```python
from build123d import *

# Parameters (mm, degrees)
BOSS_EXTRUDE1_DEPTH     = 3
CUT_EXTRUDE1_DEPTH      = 14.421065531
CUT_EXTRUDE1_DEPTH_BACK = 14.421065531
SKETCH2_R               = 1.75
SKETCH3_R               = 4
CUT_EXTRUDE2_DEPTH      = 6
FILLET1_R               = 0.4
FILLET2_R               = 1
CUT_EXTRUDE3_DEPTH      = 15.391838135
CUT_EXTRUDE3_DEPTH_BACK = 15.391838135
SKETCH4_W               = 19
SKETCH4_H               = 0.4


with BuildPart() as part:
    # Sketch1 → Boss-Extrude1 (new, symmetric)
    with BuildSketch(Plane(origin=(0, 0, 0), x_dir=(1, 0, 0), z_dir=(0, 1, 0))):
        with BuildLine():
            Line((-4.05, 0), (-9.25, 0))
            ThreePointArc((-9.25, 0), (0, 9.25), (9.25, 0))
            Line((9.25, 0), (4.05, 0))
            ThreePointArc((4.05, 0), (0, 4.05), (-4.05, 0))
        make_face()
    extrude(amount=BOSS_EXTRUDE1_DEPTH, both=True)

    # Sketch2 → Cut-Extrude1 (cut, two sides: drawn at the far end of the back side and taken through both)
    with BuildSketch(Plane.XY.offset(-CUT_EXTRUDE1_DEPTH_BACK)):
        with Locations((6.65, 0)):
            Circle(SKETCH2_R)
        with Locations((-6.65, 0)):
            Circle(SKETCH2_R)
    extrude(amount=CUT_EXTRUDE1_DEPTH + CUT_EXTRUDE1_DEPTH_BACK, mode=Mode.SUBTRACT)

    # Sketch3 → Cut-Extrude2 (cut)
    with BuildSketch(Plane.XY.offset(-10)):
        with Locations((6.65, 0)):
            Circle(SKETCH3_R)
        with Locations((-6.65, 0)):
            Circle(SKETCH3_R)
    extrude(amount=CUT_EXTRUDE2_DEPTH, mode=Mode.SUBTRACT)

    # Fillet1
    # the kernel refuses this fillet: 0.4 mm, written as the material it takes off along each edge
    with BuildSketch(Plane(origin=(-4.004248689, 3, -4), x_dir=(0.6743792283231849, -0.7383851680567708, 0), z_dir=(0, 0, -1)), Plane(origin=(4.004248689, -3, -4), x_dir=(-0.6743792283231826, 0.7383851680567729, 0), z_dir=(0, 0, -1))) as fillet1_piece_1:
        with BuildLine():
            CenterArc((0.904923131, -0.397672121), FILLET1_R, 96.184415635, 126.22154662)
            Line((0.609569064, -0.667423812), (0, 0))
            ThreePointArc((0, 0), (0.430915777, -0.023278789), (0.861831553, 0))
        make_face()
    extrude(amount=6.598116085, mode=Mode.SUBTRACT)
    with BuildSketch(Plane(origin=(-4.004248689, -3, -4), x_dir=(0.6743792283231809, 0.7383851680567743, 0), z_dir=(0, 0, -1)), Plane(origin=(4.004248689, 3, -4), x_dir=(-0.6743792283231826, -0.7383851680567729, 0), z_dir=(0, 0, -1))) as fillet1_piece_2:
        with BuildLine():
            CenterArc((0.904923131, 0.397672121), FILLET1_R, 137.594037745, 126.22154662)
            Line((0.609569064, 0.667423812), (0, 0))
            ThreePointArc((0, 0), (0.430915777, 0.023278789), (0.861831553, 0))
        make_face()
    extrude(amount=6.598116085, mode=Mode.SUBTRACT)

    # Fillet2
    # the kernel refuses this fillet: 1 mm, written as the material it adds along each edge
    with BuildSketch(Plane(origin=(-6.65, 0, -4), x_dir=(0.8067381522408935, -0.5909090909090408, 0), z_dir=(-0.5909090909090408, -0.8067381522408935, 0))) as fillet2_piece_1:
        with BuildLine():
            CenterArc((4 - FILLET2_R, -FILLET2_R), FILLET2_R, 0, 90)
            Line((4, -FILLET2_R), (4, 0))
            Line((4, 0), (4 - FILLET2_R, 0))
        make_face()
    revolve(axis=Axis((-6.65, 0, -4), (0, 0, 1)), revolution_arc=72.44309324)
    with BuildSketch(Plane(origin=(6.65, 0, -4), x_dir=(-0.8067381522408924, 0.5909090909090423, 0), z_dir=(0.5909090909090423, 0.8067381522408924, 0))) as fillet2_piece_2:
        with BuildLine():
            CenterArc((4 - FILLET2_R, -FILLET2_R), FILLET2_R, 0, 90)
            Line((4, -FILLET2_R), (4, 0))
            Line((4, 0), (4 - FILLET2_R, 0))
        make_face()
    revolve(axis=Axis((6.65, 0, -4), (0, 0, 1)), revolution_arc=72.44309324)
    with BuildSketch(Plane(origin=(-3.10035213, 2.6, -4), x_dir=(-0.8067381522410291, -0.5909090909088556, 0), z_dir=(0.5909090909088556, -0.8067381522410291, 0))) as fillet2_piece_3_section:
        with BuildLine():
            CenterArc((0.4 + FILLET2_R, FILLET2_R), FILLET2_R, 180, 90)
            Line((0.4, FILLET2_R), (0.4, 0))
            Line((0.4, 0), (0.4 + FILLET2_R, 0))
        make_face()
    fillet2_piece_3 = revolve(axis=Axis((-3.10035213, 2.6, -4), (0, 0, -1)), revolution_arc=359.64, mode=Mode.PRIVATE)
    fillet2_piece_3 = split(fillet2_piece_3, bisect_by=Plane(origin=(-3.794786047, 3, -4.154806291), z_dir=(0, -1, 0)), keep=Keep.TOP, mode=Mode.PRIVATE)
    add(fillet2_piece_3)
    with BuildSketch(Plane(origin=(-3.10035213, -2.6, -4), x_dir=(-0.8030094610318433, 0.5959662788223411, 0), z_dir=(-0.5959662788223411, -0.8030094610318433, 0))) as fillet2_piece_4_section:
        with BuildLine():
            CenterArc((-0.4 - FILLET2_R, FILLET2_R), FILLET2_R, 270, 90)
            Line((-0.4 - FILLET2_R, 0), (-0.4, 0))
            Line((-0.4, 0), (-0.4, FILLET2_R))
        make_face()
    fillet2_piece_4 = revolve(axis=Axis((-3.10035213, -2.6, -4), (0, 0, -1)), revolution_arc=359.64, mode=Mode.PRIVATE)
    fillet2_piece_4 = split(fillet2_piece_4, bisect_by=Plane(origin=(-3.549155049, -3, -4.290205519), z_dir=(0, 1, 0)), keep=Keep.TOP, mode=Mode.PRIVATE)
    add(fillet2_piece_4)
    with BuildSketch(Plane(origin=(3.10035213, -2.6, -4), x_dir=(0.8067381522410291, 0.5909090909088556, 0), z_dir=(-0.5909090909088556, 0.8067381522410291, 0))) as fillet2_piece_5_section:
        with BuildLine():
            CenterArc((0.4 + FILLET2_R, FILLET2_R), FILLET2_R, 180, 90)
            Line((0.4, FILLET2_R), (0.4, 0))
            Line((0.4, 0), (0.4 + FILLET2_R, 0))
        make_face()
    fillet2_piece_5 = revolve(axis=Axis((3.10035213, -2.6, -4), (0, 0, -1)), revolution_arc=359.64, mode=Mode.PRIVATE)
    fillet2_piece_5 = split(fillet2_piece_5, bisect_by=Plane(origin=(3.794786054, -3, -4.154806275), z_dir=(0, 1, 0)), keep=Keep.TOP, mode=Mode.PRIVATE)
    add(fillet2_piece_5)
    with BuildSketch(Plane(origin=(3.10035213, 2.6, -4), x_dir=(0.8030094610318433, -0.5959662788223411, 0), z_dir=(0.5959662788223411, 0.8030094610318433, 0))) as fillet2_piece_6_section:
        with BuildLine():
            CenterArc((-0.4 - FILLET2_R, FILLET2_R), FILLET2_R, 270, 90)
            Line((-0.4, FILLET2_R), (-0.4, 0))
            Line((-0.4, 0), (-0.4 - FILLET2_R, 0))
        make_face()
    fillet2_piece_6 = revolve(axis=Axis((3.10035213, 2.6, -4), (0, 0, -1)), revolution_arc=359.64, mode=Mode.PRIVATE)
    fillet2_piece_6 = split(fillet2_piece_6, bisect_by=Plane(origin=(3.549155046, 3, -4.290205778), z_dir=(0, -1, 0)), keep=Keep.TOP, mode=Mode.PRIVATE)
    add(fillet2_piece_6)

    # Sketch4 → Cut-Extrude3 (cut, two sides: drawn at the far end of the back side and taken through both)
    with BuildSketch(Plane(origin=(0, 3, 0), x_dir=(1, 0, 0), z_dir=(0, 1, 0)).offset(-CUT_EXTRUDE3_DEPTH_BACK)):
        Rectangle(SKETCH4_W, SKETCH4_H)
    extrude(amount=CUT_EXTRUDE3_DEPTH + CUT_EXTRUDE3_DEPTH_BACK, mode=Mode.SUBTRACT)


solid = part.part
```
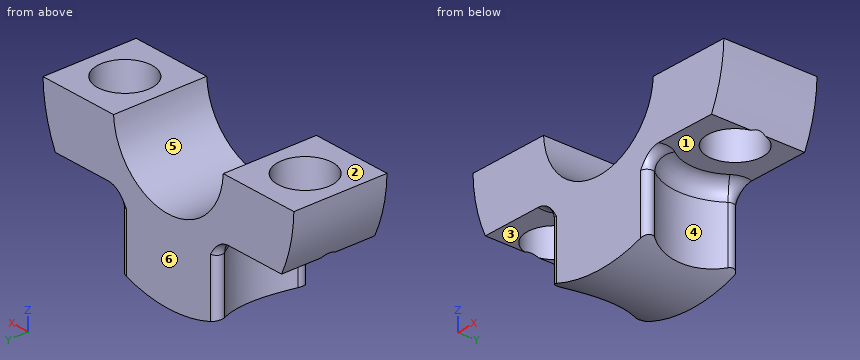
CAD build for the part. Positions are in the model's coordinates, mm. Face numbers are marked on the shaded views. A direction names the side the tool comes from. Coordinates: 2 decimals unless noted, no trailing zeros. Write each loop counter-clockwise with the first axis right and the second up, starting at its lowest first coordinate (ties: lowest second). Pieces come first, ordered by that corner, then holes.
(1) Cut at D-D, the plane z = -4.75. List the corners of the cut face in (x, y), and give its area (3 significant figures).
(2) Two-plate mould, pull along Y, no slides. Class the marked faces 4, 5 and 6: +Y half, -Y half, draft (parallel to the pull), parting line (faces both ways), or undercut.
(3) 3-axis set-ups, long thin cutter, end or side, ignore diameter. For the marked faces 1, 2 and 3: which of +Z, -Z, +X, -X, +Y, -Y reach the whole face in a straight line?
(4) Cut at A-A, the plane x = 6.65. List the corners of the cut face in (y, z), and give its area (3 significant figures).
(5) Cut at C-C, the plane z = -1. List the corners of the cut face in (x, y).
(6) Drill centre lines: probe 1 along Y at (x, z) = (6.65, -2.5); probe 2 along X at (y, z) = (0, -1.9); probe 3 along X at (y, z) = (0, -2.3). Where is each one in solid material? Low to high.
(7) Flat gauge pins, fed straight in: pin 1 (1.4 mm diameter, centred on x = 5, y = -0.5, fed in from -Z); pin 2 (1.5 mm diameter, centred on y = -1, z = -7.5, fed in from +X). Where does each tip first touch, or does it go through?
Geometry says:
1. outline: (-3.45, -2.34) arc R0.43 ccw to (-3.26, -3) - (3.26, -3) arc R0.43 ccw to (3.45, -2.34) arc R3.97 cw to (3.45, 2.34) arc R0.43 ccw to (3.26, 3) - (-3.26, 3) arc R0.43 ccw to (-3.45, 2.34) arc R3.97 cw to start
1. area: 36.6 mm2
2. face 4: undercut
2. face 5: draft
2. face 6: +Y half
3. face 1: -Z, +X
3. face 2: +Z, +X, -X, +Y, -Y
3. face 3: -Z, -X
4. outline: (-3, -4) - (-1.75, -4) - (-1.75, -0.2) - (-3, -0.2) - close; (1.75, -4) - (3, -4) - (3, -0.2) - (1.75, -0.2) - close
4. area: 9.50 mm2
5. outline: (-9.2, -3) - (-3.92, -3) - (-3.92, 3) - (-9.2, 3) - close; (3.92, -3) - (9.2, -3) - (9.2, 3) - (3.92, 3) - close; hole circle Ø3.5 at (-6.65, 0); hole circle Ø3.5 at (6.65, 0)
6. probe 1: y = -3 to -1.75, 1.75 to 3
6. probe 2: x = -9.05 to -8.4, -4.9 to -3.58, 3.58 to 4.9, 8.4 to 9.05
6. probe 3: x = -8.96 to -8.4, -4.9 to -3.33, 3.33 to 4.9, 8.4 to 8.96
7. pin 1: stops at z = -4
7. pin 2: stops at x = 3.05
